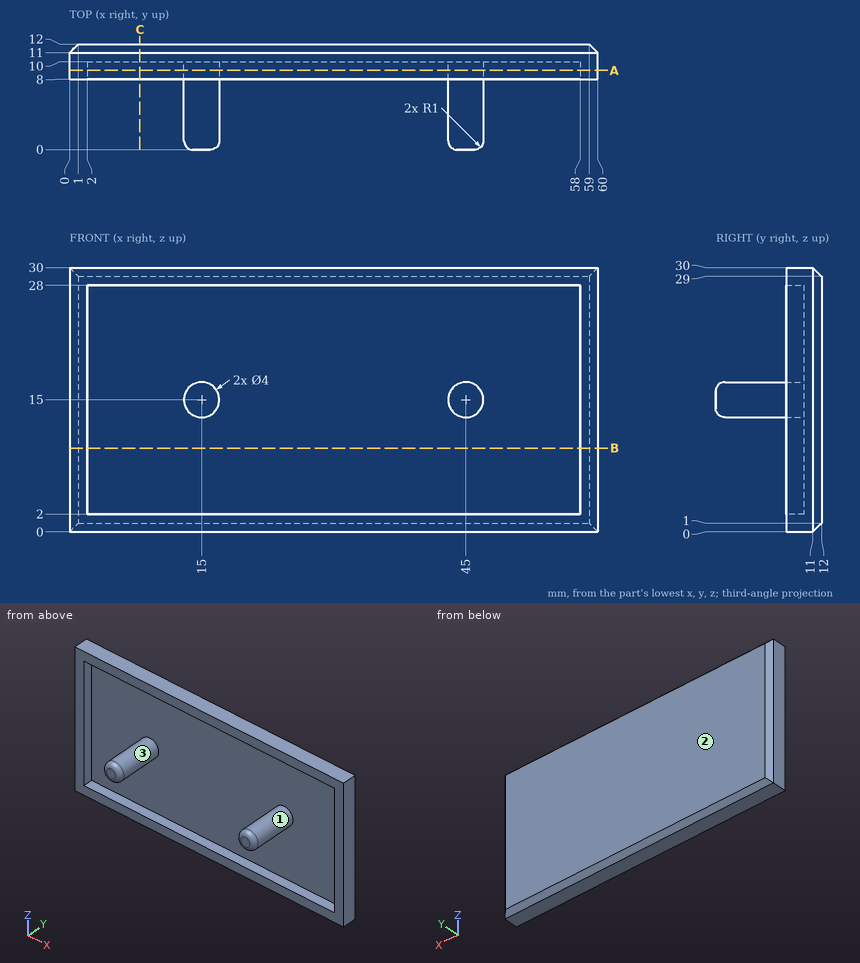
Study the drawing (mm; zero at the part's minimum x, y, z) and answer. Coordinates: 2 decimals unless noted, no trailing zeros. Order: outer loops, then holes, each group sorted by start corner. A loop starts at its lowest first (then second) coordinate and runs counter-clockwise, first axis right, second up. Notation, with made-up numbers: (-24, 66) -> (32, 66) arc R14 cw to (32, 91) -> close; hole circle Ø1 at (69, -1.5). An arc over 180 degrees is marked (long way). Answer in a Markdown table with one row per item. Add a question column.
Item 1: Find section A-A (y = 9). Write down the section's boundary in (x, z), then the cut area to 3 significant figures.
Item 2: Find the intervals of material crossed by L1, parallel to X at y = 9.5, z = 26.5; L2, parallel to Z at x = 16.5, y = 9.75; L3, parallel to Y at x = 43.5, z = 3, in increasing order. Write a range as from..to.
Item 3: Find section C-C (x = 8). Write down the section's boundary in (y, z).
Item 4: Each of these flat-tipped pins is pushed along its axis until it touches: P1, Ø1.6, axis at x = 32.5, y = 8.5, coming from the -Z side; P2, Ø5, axis at y = 2, z = 15, coming from the -X side; P3, Ø13, axis at x = 32, z = 9, coming from the -Y side; P4, Ø4, axis at x = 44, y = 4.5, coming from the -Z side. Where does it stop, or does it pass through?
Item 5: Find section B-B (z = 9.5). Write down the section's boundary in (x, y), then the cut area to 3 significant figures.
Item 6: Determine the mould class of the marked faces 1, 2 and 3 for opening direction Z: +Z half, -Z half, draft (parallel to the pull), parting line (faces both ways), or undercut.
Result set:
| question | item | result |
|---|---|---|
| 1 | outline | (0, 0) -> (60, 0) -> (60, 30) -> (0, 30) -> close; circle Ø4 at (15, 15); circle Ø4 at (45, 15); hole (2, 2) -> (58, 2) -> (58, 28) -> (2, 28) -> close |
| 1 | area | 369 mm² |
| 2 | L1 | x = 0..2, 58..60 |
| 2 | L2 | z = 0..2, 13.68..16.32, 28..30 |
| 2 | L3 | y = 10..12 |
| 3 | outline | (8, 0) -> (11, 0) -> (12, 1) -> (12, 29) -> (11, 30) -> (8, 30) -> (8, 28) -> (10, 28) -> (10, 2) -> (8, 2) -> close |
| 4 | P1 | stops at z = 0 |
| 4 | P2 | stops at x = 13 |
| 4 | P3 | stops at y = 10 |
| 4 | P4 | stops at z = 13 |
| 5 | outline | (0, 8) -> (2, 8) -> (2, 10) -> (58, 10) -> (58, 8) -> (60, 8) -> (60, 11) -> (59, 12) -> (1, 12) -> (0, 11) -> close |
| 5 | area | 127 mm² |
| 6 | face 1 | undercut |
| 6 | face 2 | draft |
| 6 | face 3 | undercut |
